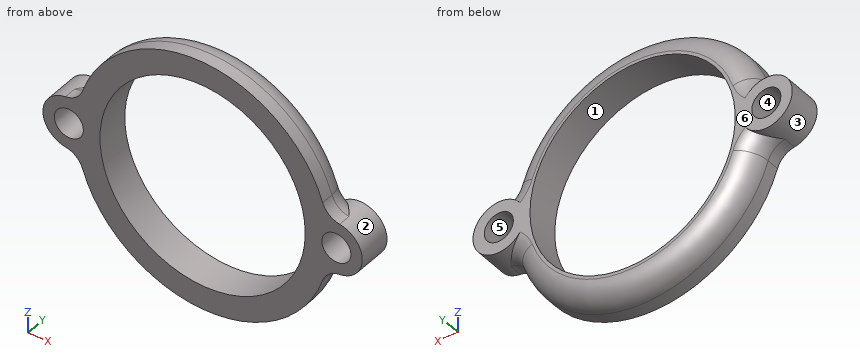
```python
from build123d import *

# Parameters (mm, degrees)
F0_R     = 24.75
F1_DEPTH = 8
F3_R     = 5
F2_R     = 6.25
F2_R_2   = 3.5
F4_DEPTH = 8


with BuildPart() as f1:
    # F0 (on Front) → F1 (new body)
    with BuildSketch(Plane.XZ):
        with BuildLine():
            ThreePointArc((33.056416882, 6.1977569985), (30.5178723488, 7.3005515757), (28.9548531499, 9.5847002596))
            ThreePointArc((28.9548531499, 9.5847002596), (0, 30.5), (-28.9548531499, 9.5847002596))
            ThreePointArc((-28.9548531499, 9.5847002596), (-30.5178723488, 7.3005515757), (-33.056416882, 6.1977569985))
            ThreePointArc((-33.056416882, 6.1977569985), (-28.1255367326, 4.6958814674), (-26, 0))
            ThreePointArc((-26, 0), (-28.1255367326, -4.6958814674), (-33.056416882, -6.1977569985))
            ThreePointArc((-33.056416882, -6.1977569985), (-30.5178723488, -7.3005515757), (-28.9548531499, -9.5847002596))
            ThreePointArc((-28.9548531499, -9.5847002596), (0, -30.5), (28.9548531499, -9.5847002596))
            ThreePointArc((28.9548531499, -9.5847002596), (30.5178723488, -7.3005515757), (33.056416882, -6.1977569985))
            ThreePointArc((33.056416882, -6.1977569985), (26, 0), (33.056416882, 6.1977569985))
        make_face()
        Circle(F0_R, mode=Mode.SUBTRACT)
    extrude(amount=-F1_DEPTH)

    # F3
    f3_edges = [f1.edges().sort_by_distance(p)[0] for p in [
        (30.517872, 8, -7.300552),
        (0, 8, -30.5),
        (0, 8, 30.5),
    ]]
    fillet(f3_edges, radius=F3_R)

    # F2 (on Front) → F4 (join)
    with BuildSketch(Plane.XZ):
        with Locations((32.25, 0)):
            Circle(F2_R)
        with Locations((32.25, 0)):
            Circle(F2_R_2, mode=Mode.SUBTRACT)
        with Locations((-32.25, 0)):
            Circle(F2_R)
        with Locations((-32.25, 0)):
            Circle(F2_R_2, mode=Mode.SUBTRACT)
    extrude(amount=-F4_DEPTH)


solid = f1.part
```
Here's how the part is built. I have some questions about the finished solid (model axes, mm). Face numbers are marked on the shaded views. A direction names the side the tool comes from. Round coordinates to 2 decimals unless told otherwise and drop trailing zeros. Order: outer loops, then holes, each group sorted by start corner. A loop starts at its lowest first (then second) coordinate and runs counter-clockwise, first axis right, second up. Notation, with made-up numbers: (79.25, -20) -> (94.25, -20) arc R33 cw to (94.25, 8) -> close; hole circle Ø11 at (55, -22). An arc over 180 degrees is marked (long way). Use a Markdown table: item, result. Add a question column.
(1) I need wall thicknesses on line 1 along Z through (x, y) = (32.25, 5.25); line 2 along Z through (x, y) = (20, 4.25); line 3 along X through (y, z) = (4.5, -5.5). Which ranges of each line are inside material? Lowest first, please.
(2) For the marked faces 1 and 2, which set-ups out of +Z, -Z, +X, -X, +Y, -Y let a thin tool reach every point of the face, with its end or its side?
(3) For pin 1 Ø1.5 at (x, y) = (16, 3) entering from +Z; pin 2 Ø1.5 at (y, z) = (2.5, 10.5) entering from +X, each with a flat end and sliding along its axis, tell me the tip position at first contact or that it passes through.
(4) Suppose I cut it at D-D, the plane y = 6.25. Please give me the cut outline in (x, z), and give its area (3 significant figures).
(5) Suppose I cut it at B-B, the plane y = 1.25. Please give me the cut outline in (x, z), and give its area (3 significant figures).
(6) Suppose I cut it at A-A, the plane x = 0. Please give me the cut outline in (y, z), and give its area (3 significant figures).
(7) If we mould it in two halves opening along Z, with no side actions, what happens to the marked faces 3, 4, 5 and 6? For each: released by +Z, released by -Z, zero draft, split by the parting line, or undercut.
(8) Suppose I cut it at C-C, the plane z = 0. Please give me the cut outline in (x, y), and give its area (3 significant figures).
Verdict:
| question | item | result |
|---|---|---|
| 1 | line 1 | -6.25 to -3.5, 3.5 to 6.25 |
| 1 | line 2 | -22.82 to -14.58, 14.58 to 22.82 |
| 1 | line 3 | -35.22 to -24.13, 24.13 to 35.22 |
| 2 | face 1 | +Y, -Y |
| 2 | face 2 | +Y |
| 3 | pin 1 | z = 26.41 |
| 3 | pin 2 | x = 28.9 |
| 4 | outline | (-30.33, -5.95) arc R6.2 cw to (-27.82, -9.21) arc R29.3 ccw to (27.82, -9.21) arc R6.2 cw to (30.33, -5.95) arc R6.25 ccw (long way) to (30.33, 5.95) arc R6.2 cw to (27.82, 9.21) arc R29.3 ccw to (-27.82, 9.21) arc R6.2 cw to (-30.33, 5.95) arc R6.25 ccw (long way) to start; hole circle Ø7 at (-32.25, 0); hole circle Ø49.5 at (0, 0); hole circle Ø7 at (32.25, 0) |
| 4 | area | 901 mm2 |
| 5 | outline | (-33.06, -6.2) arc R5 cw to (-28.95, -9.58) arc R30.5 ccw to (28.95, -9.58) arc R5 cw to (33.06, -6.2) arc R6.25 ccw to (33.06, 6.2) arc R5 cw to (28.95, 9.58) arc R30.5 ccw to (-28.95, 9.58) arc R5 cw to (-33.06, 6.2) arc R6.25 ccw to start; hole circle Ø7 at (-32.25, 0); hole circle Ø49.5 at (0, 0); hole circle Ø7 at (32.25, 0) |
| 5 | area | 1,100 mm2 |
| 6 | outline | (0, -30.5) -> (3, -30.5) arc R5 ccw to (8, -25.5) -> (8, -24.75) -> (0, -24.75) -> close; (0, 24.75) -> (8, 24.75) -> (8, 25.5) arc R5 ccw to (3, 30.5) -> (0, 30.5) -> close |
| 6 | area | 81.3 mm2 |
| 7 | face 3 | split by the parting line |
| 7 | face 4 | undercut |
| 7 | face 5 | undercut |
| 7 | face 6 | zero draft |
| 8 | outline | (-38.5, 0) -> (-35.75, 0) -> (-35.75, 8) -> (-38.5, 8) -> close; (-28.75, 0) -> (-24.75, 0) -> (-24.75, 8) -> (-28.75, 8) -> close; (24.75, 0) -> (28.75, 0) -> (28.75, 8) -> (24.75, 8) -> close; (35.75, 0) -> (38.5, 0) -> (38.5, 8) -> (35.75, 8) -> close |
| 8 | area | 108 mm2 |
